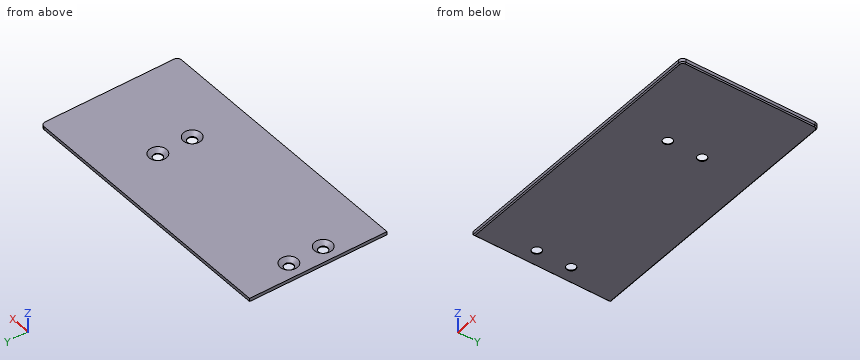
```python
from build123d import *

# Parameters (mm, degrees)
SKETCH1_W                                   = 202.40625
SKETCH1_H                                   = 3.175
BOSS_EXTRUDE1_DEPTH                         = 101.6
CSK_FOR_1_4_FLAT_HEAD_MACHINE_SCREW_2_COUNT = 2
CSK_FOR_1_4_FLAT_HEAD_MACHINE_SCREW_2_PITCH = 25.4
CSK_FOR_1_4_FLAT_HEAD_MACHINE_SCREW_3_COUNT = 2
CSK_FOR_1_4_FLAT_HEAD_MACHINE_SCREW_3_PITCH = 129.515095645
CSK_FOR_1_4_FLAT_HEAD_MACHINE_SCREW_4_COUNT = 2
CSK_FOR_1_4_FLAT_HEAD_MACHINE_SCREW_4_PITCH = 127
CUT_EXTRUDE1_DEPTH                          = 4.175
CHAMFER1_SIZE                               = 0.7874


with BuildPart() as part:
    # Sketch1 → Boss-Extrude1 (new body)
    with BuildSketch(Plane(origin=(0, 0, 0), x_dir=(1, 0, 0), z_dir=(0, 1, 0))):
        with Locations((101.203125, -1.5875)):
            Rectangle(SKETCH1_W, SKETCH1_H)
    extrude(amount=-BOSS_EXTRUDE1_DEPTH)

    # Sketch15 → CSK for 1/4 Flat Head Machine Screw (100)5 (revolve, cut)
    with BuildSketch(Plane(origin=(11.90625, -38.1, 3.175), x_dir=(0, -1, 0), z_dir=(1, 0, 0))):
        Polygon((0, 0), (0, 3.175), (3.3782, 3.175), (3.3782, 2.568232241), (6.4389, 0), align=None)
    csk_for_1_4_flat_head_machine_screw_100 = revolve(axis=Axis((11.90625, -38.1, 9.525), (0, 0, -1)), mode=Mode.SUBTRACT)

    # CSK for 1_4 Flat Head Machine Screw  2: CSK for 1/4 Flat Head Machine Screw (100)5 ×2
    with Locations(*[(0, -i * CSK_FOR_1_4_FLAT_HEAD_MACHINE_SCREW_2_PITCH, 0) for i in range(1, CSK_FOR_1_4_FLAT_HEAD_MACHINE_SCREW_2_COUNT)]):
        add(csk_for_1_4_flat_head_machine_screw_100, mode=Mode.SUBTRACT)

    # CSK for 1_4 Flat Head Machine Screw  3: CSK for 1/4 Flat Head Machine Screw (100)5 ×2
    with Locations(*[Vector(0.980580676, -0.196116135, 0) * (i * CSK_FOR_1_4_FLAT_HEAD_MACHINE_SCREW_3_PITCH) for i in range(1, CSK_FOR_1_4_FLAT_HEAD_MACHINE_SCREW_3_COUNT)]):
        add(csk_for_1_4_flat_head_machine_screw_100, mode=Mode.SUBTRACT)

    # CSK for 1_4 Flat Head Machine Screw  4: CSK for 1/4 Flat Head Machine Screw (100)5 ×2
    with Locations(*[(i * CSK_FOR_1_4_FLAT_HEAD_MACHINE_SCREW_4_PITCH, 0, 0) for i in range(1, CSK_FOR_1_4_FLAT_HEAD_MACHINE_SCREW_4_COUNT)]):
        add(csk_for_1_4_flat_head_machine_screw_100, mode=Mode.SUBTRACT)

    # Sketch17 → Cut-Extrude1 (cut, through all)
    with BuildSketch(Plane.XY.offset(3.175)):
        with BuildLine():
            Line((202.40625, -3.175), (202.40625, 0))
            Line((202.40625, 0), (199.23125, 0))
            ThreePointArc((199.23125, 0), (201.47631403, -0.92993597), (202.40625, -3.175))
        make_face()
        with BuildLine():
            Line((202.40625, -98.425), (202.40625, -101.6))
            Line((202.40625, -101.6), (199.23125, -101.6))
            ThreePointArc((199.23125, -101.6), (201.47631403, -100.67006403), (202.40625, -98.425))
        make_face()
    extrude(amount=-CUT_EXTRUDE1_DEPTH, mode=Mode.SUBTRACT)

    # Chamfer1
    chamfer1_edges = [part.edges().sort_by_distance(p)[0] for p in [
        (99.615625, 0, 0),
        (99.615625, -101.6, 0),
        (202.40625, -50.8, 0),
        (201.47631403, -0.92993597, 0),
        (201.47631403, -100.67006403, 0),
        (0, -50.8, 0),
    ]]
    chamfer(chamfer1_edges, length=CHAMFER1_SIZE)


solid = part.part
```
Can you work these out from the model? Positions are in its coordinate system, mm. Coordinates: 2 decimals unless noted, no trailing zeros. Loops run counter-clockwise (first coordinate to the right, second up) from the corner with the lowest first, then second, coordinate; pieces in that order, holes last.
1) Imagine slicing it at B-B on z = 2.6. List the corners of the cut face in (x, y) for me (3 decimals).
2) I need wall thicknesses on probe 1 along X at (y, z) = (-38.1, 0.45); probe 2 along X at (y, z) = (-40, 1.7); probe 3 along Y at (x, z) = (157.5, 0.7). Which ranges of each line are inside material? Lowest first, please.
3) For pin 1 (11 mm diameter, centred on x = 138.91, y = -63.5, fed in from +Z), with a flat end and sliding along its axis, tell me the tip position at first contact or that it passes through.
4) Imagine slicing it at A-A on y = -38.1. List the corners of the cut face in (x, z) for me (3 decimals), plus the area to 3 significant figures.
Completed:
1. outline: (0, -101.6) - (199.231, -101.6) arc R3.175 ccw to (202.406, -98.425) - (202.406, -3.175) arc R3.175 ccw to (199.231, 0) - (0, 0) - close; hole circle Ø11.507 at (11.906, -63.5); hole circle Ø11.507 at (11.906, -38.1); hole circle Ø11.507 at (138.906, -63.5); hole circle Ø11.507 at (138.906, -38.1)
2. probe 1: x = 0.34 to 8.53, 15.28 to 135.53, 142.28 to 202.07
2. probe 2: x = 0 to 7.63, 16.18 to 134.63, 143.18 to 202.41
2. probe 3: y = -101.51 to -0.09
3. pin 1: stops at z = 2.39
4. outline: (0, 0.787) - (0.787, 0) - (8.528, 0) - (8.528, 0.607) - (5.467, 3.175) - (0, 3.175) - close; (15.284, 0) - (135.528, 0) - (135.528, 0.607) - (132.467, 3.175) - (18.345, 3.175) - (15.284, 0.607) - close; (142.284, 0) - (201.619, 0) - (202.406, 0.787) - (202.406, 3.175) - (145.345, 3.175) - (142.284, 0.607) - close
4. area: 583 mm2
